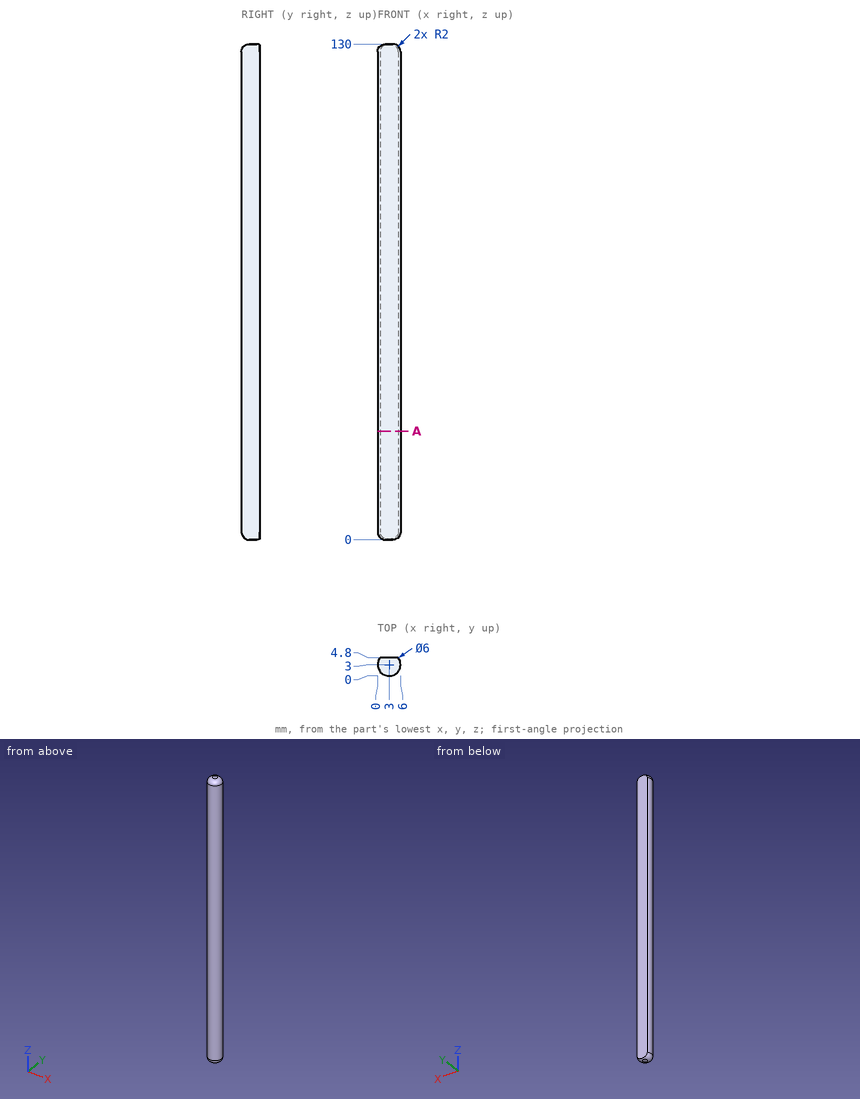
Study the drawing (mm; zero at the part's minimum x, y, z) and answer. Round coordinates to 2 decimals unless told otherwise and drop trailing zeros. Write each loop counter-clockwise with the first axis right and the second up, starting at its lowest first coordinate (ties: lowest second). Pieces come first, ordered by that corner, then holes. Notation, with made-up numbers: (-19.75, 74.25) - (-10.75, 74.25) arc R32 ccw to (-10.75, 107.25) - close; hole circle Ø5 at (-25.75, 41). An arc over 180 degrees is marked (long way). Use a Markdown table: item, result. Add a question column.
1. Consider line 1 (X direction, y = 3.15, z = 61.5); line 2 (Y direction, x = 2.75, z = 66.5); line 3 (Y direction, x = 4, z = 80). Determine where each line is inside the solid, lowest interval first.
2. The part is cut by section A-A (z = 28.5). Write down the section's boundary in (x, y), and give its area (3 significant figures).
3. A flat-ended cylindrical pin translates along its axis: P1, Ø1, axis at y = 2, z = 42, coming from the +X side. Find the tip coordinate at first contact, or state that the pin passes through.
Reported:
| question | item | result |
|---|---|---|
| 1 | line 1 | 0 to 6 |
| 1 | line 2 | 0.01 to 4.8 |
| 1 | line 3 | 0.17 to 4.8 |
| 2 | outline | (0.6, 4.8) arc R3 ccw (long way) to (5.4, 4.8) - close |
| 2 | area | 24.2 mm^2 |
| 3 | P1 | x = 5.96 |
